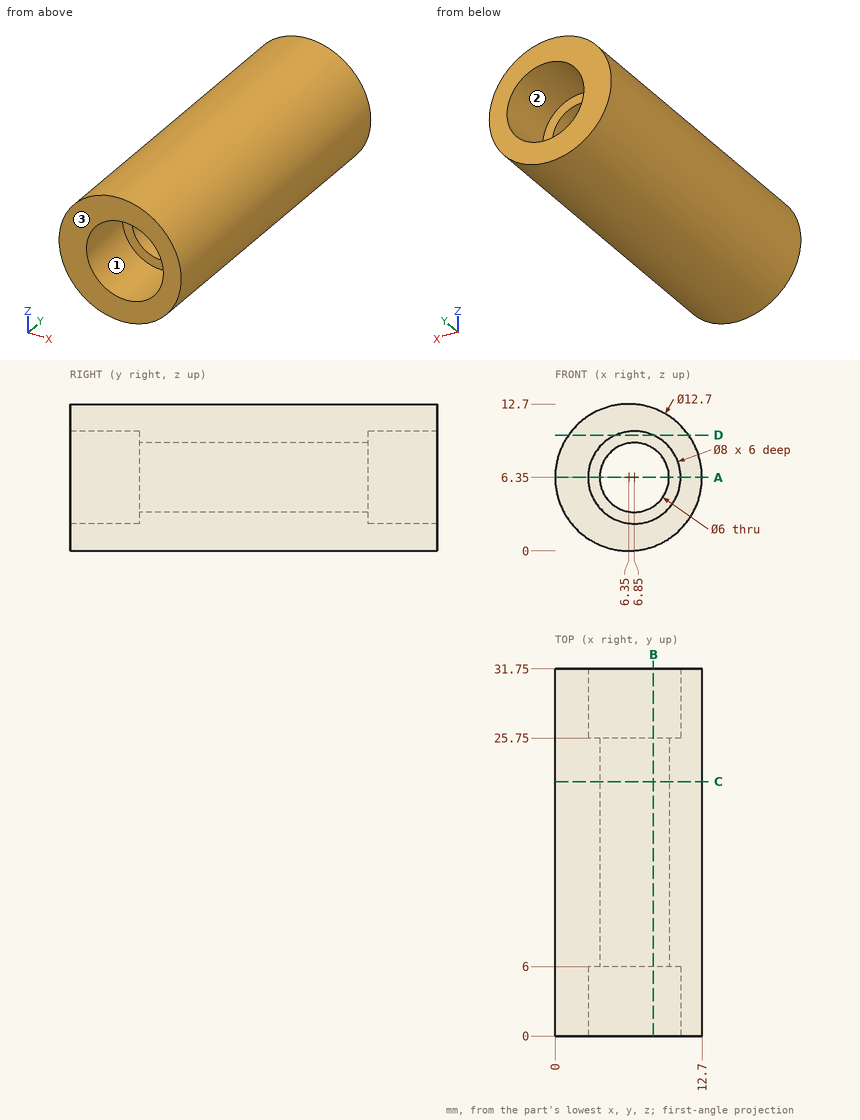
The figure shows three views and two pictorial views of one solid part (mm, origin at its lowest corner). Answer the questions. A direction names the side the tool comes from. Coordinates: 2 decimals unless noted, no trailing zeros. Write each loop counter-clockwise with the first axis right and the second up, starting at its lowest first coordinate (ties: lowest second). Pieces come first, ordered by that corner, then holes. Notation, with made-up numbers: (72, 25.5) -> (88, 25.5) arc R9 ccw to (88, 31.5) -> close; hole circle Ø6 at (75, 89). An arc over 180 degrees is marked (long way). Return JSON: item names as keys, results as strings.
(1) The part is cut by section B-B on x = 8.5. Give the vertices of the cut face in (y, z), then the cut area to 3 significant figures.
Answers below:
{"outline": "(0, 0.38) -> (31.75, 0.38) -> (31.75, 2.71) -> (25.75, 2.71) -> (25.75, 3.84) -> (6, 3.84) -> (6, 2.71) -> (0, 2.71) -> close; (0, 9.99) -> (6, 9.99) -> (6, 8.86) -> (25.75, 8.86) -> (25.75, 9.99) -> (31.75, 9.99) -> (31.75, 12.32) -> (0, 12.32) -> close", "area": "193 mm^2"}
(2) The part is cut by section D-D on z = 10. Give the vertices of the cut face in (x, y).
Answers below:
{"outline": "(1.15, 0) -> (5.21, 0) -> (5.21, 6) -> (8.49, 6) -> (8.49, 0) -> (11.55, 0) -> (11.55, 31.75) -> (8.49, 31.75) -> (8.49, 25.75) -> (5.21, 25.75) -> (5.21, 31.75) -> (1.15, 31.75) -> close"}
(3) Each of these flat-tipped pins is pushed along its axis until it touches: P1, Ø6, axis at y = 26, z = 9, coming from the -X side; P2, Ø2.5, axis at x = 5.5, z = 5, coming from the +Y side; P3, Ø4, axis at y = 6.5, z = 11, coming from the +X side; P4, Ø4, axis at y = 20, z = 3.5, coming from the +X side. Where does it stop, or does it pass through?
Answers below:
{"P1": "x = 0", "P2": "y = 25.75", "P3": "x = 12.12", "P4": "x = 12.64"}
(4) Which of the six approach directions +Z, -Z, +X, -X, +Y, -Y give full straight-line access (tool end or side, diameter ignored) to the marked faces 1, 2 and 3?
Answers below:
{"face 1": "-Y", "face 2": "+Y", "face 3": "+Z, -Z, +X, -X, -Y"}
(5) The part is cut by section C-C on y = 22. Give the vertices of the cut face in (x, z).
Answers below:
{"outline": "circle Ø12.7 at (6.35, 6.35); hole circle Ø6 at (6.85, 6.35)"}
(6) Consider line 1 along Z through (x, y) = (6.85, 12.5); line 2 along X through (y, z) = (4, 6.5); line 3 along Z through (x, y) = (6.85, 1.3). Determine where each line is inside the solid, lowest interval first. Write a range as from..to.
Answers below:
{"line 1": "0.02..3.35, 9.35..12.68", "line 2": "0..2.85, 10.85..12.7", "line 3": "0.02..2.35, 10.35..12.68"}
(7) The part is cut by section A-A on z = 6.35. Give the vertices of the cut face in (x, y), then the cut area to 3 significant figures.
Answers below:
{"outline": "(0, 0) -> (2.85, 0) -> (2.85, 6) -> (3.85, 6) -> (3.85, 25.75) -> (2.85, 25.75) -> (2.85, 31.75) -> (0, 31.75) -> close; (9.85, 6) -> (10.85, 6) -> (10.85, 0) -> (12.7, 0) -> (12.7, 31.75) -> (10.85, 31.75) -> (10.85, 25.75) -> (9.85, 25.75) -> close", "area": "189 mm^2"}
